The listing builds one solid part. Answer for the finished solid, in the listing's coordinates (mm). A direction names the side the tool comes from. Coordinates: 2 decimals unless noted, no trailing zeros. Order: outer loops, then holes, each group sorted by start corner. A loop starts at its lowest first (then second) coordinate and runs counter-clockwise, first axis right, second up.
```python
from build123d import *

# Parameters (mm, degrees)
BOSS_EXTRUDE1_DEPTH = 139
SKETCH5_R           = 2
CUT_EXTRUDE1_DEPTH  = 148.549991528
SKETCH6_W           = 3
SKETCH6_H           = 35
BOSS_EXTRUDE2_DEPTH = 35
SKETCH7_W           = 133
SKETCH7_H           = 35
BOSS_EXTRUDE3_DEPTH = 5
SKETCH8_W           = 133
SKETCH8_H           = 35
CUT_EXTRUDE2_DEPTH  = 20
SKETCH9_W           = 3
SKETCH9_H           = 12
BOSS_EXTRUDE4_DEPTH = 25
SKETCH10_W          = 133
SKETCH10_H          = 50
BOSS_EXTRUDE5_DEPTH = 20
SKETCH11_W          = 139
SKETCH11_H          = 53
CUT_EXTRUDE3_DEPTH  = 20


with BuildPart() as part:
    # Sketch3 → Boss-Extrude1 (new body)
    with BuildSketch(Plane(origin=(0, 0, 0), x_dir=(0, 0, -1), z_dir=(1, 0, 0))):
        Polygon((-34.8080918, 35), (-34.8080918, 10), (-22.8080918, 10), (-22.8080918, 35), (-19.8080918, 35), (-19.8080918, 0), (15.1919082, 0), (15.1919082, -3), (-29.8080918, -3), (-37.8080918, -3), (-37.8080918, 0), (-37.8080918, 35), align=None)
    extrude(amount=BOSS_EXTRUDE1_DEPTH)

    # Sketch5 → Cut-Extrude1 (cut, through all)
    with BuildSketch(Plane(origin=(0, 0, 19.8080918), x_dir=(-1, 0, 0), z_dir=(0, 0, -1))):
        with Locations(Location((-119, 30, 0), (0, 0, 90))):
            Circle(SKETCH5_R)
        with BuildLine():
            Line((-85, 32), (-15, 32))
            ThreePointArc((-15, 32), (-13, 30), (-15, 28))
            Line((-15, 28), (-85, 28))
            ThreePointArc((-85, 28), (-87, 30), (-85, 32))
        make_face()
    extrude(amount=-CUT_EXTRUDE1_DEPTH, mode=Mode.SUBTRACT)

    # Sketch6 → Boss-Extrude2 (add)
    with BuildSketch(Plane(origin=(0, 0, 0), x_dir=(1, 0, 0), z_dir=(0, 1, 0))):
        with Locations((1.5, -2.3080918)):
            Rectangle(SKETCH6_W, SKETCH6_H)
        with Locations((137.5, -2.3080918)):
            Rectangle(SKETCH6_W, SKETCH6_H)
    extrude(amount=BOSS_EXTRUDE2_DEPTH)

    # Sketch7 → Boss-Extrude3 (add)
    with BuildSketch(Plane(origin=(0, 0, 19.8080918), x_dir=(-1, 0, 0), z_dir=(0, 0, -1))):
        with Locations((-69.5, 17.5)):
            Rectangle(SKETCH7_W, SKETCH7_H)
    extrude(amount=BOSS_EXTRUDE3_DEPTH)

    # Sketch8 → Cut-Extrude2 (cut)
    with BuildSketch(Plane(origin=(0, 0, 14.8080918), x_dir=(-1, 0, 0), z_dir=(0, 0, -1))):
        with Locations((-69.5, 17.5)):
            Rectangle(SKETCH8_W, SKETCH8_H)
    extrude(amount=-CUT_EXTRUDE2_DEPTH, mode=Mode.SUBTRACT)

    # Sketch9 → Boss-Extrude4 (add)
    with BuildSketch(Plane(origin=(0, 10, 0), x_dir=(1, 0, 0), z_dir=(0, 1, 0))):
        with Locations((137.5, -28.8080918)):
            Rectangle(SKETCH9_W, SKETCH9_H)
        with Locations((1.5, -28.8080918)):
            Rectangle(SKETCH9_W, SKETCH9_H)
    extrude(amount=BOSS_EXTRUDE4_DEPTH)

    # Sketch10 → Boss-Extrude5 (add)
    with BuildSketch(Plane(origin=(0, 0, 0), x_dir=(1, 0, 0), z_dir=(0, 1, 0))):
        with Locations((69.5, -9.8080918)):
            Rectangle(SKETCH10_W, SKETCH10_H)
    extrude(amount=BOSS_EXTRUDE5_DEPTH)

    # Sketch11 → Cut-Extrude3 (cut)
    with BuildSketch(Plane.XZ.offset(3)):
        with Locations((69.5, 11.3080918)):
            Rectangle(SKETCH11_W, SKETCH11_H)
    extrude(amount=-CUT_EXTRUDE3_DEPTH, mode=Mode.SUBTRACT)


solid = part.part
```
1) The mould has two halves that part along X. Classify faces 1 (the flat face through (136, 27, 10)), 2 (the flat face through (0, 26, 12)), 3 (the flat face through (139, 26, 12)), 4 (the flat face through (69, 26, 37.808)): released by +X, released by -X, zero draft, split by the parting line, or undercut.
2) Each of these flat-tipped pins is pushed along its axis until it touches: P1, Ø3.5, axis at x = 119, y = 30, coming from the +Z side; P2, Ø2, axis at x = 86, y = 28.5, coming from the -Z side. Where does it stop, or does it pass through?
3) A cutting plane is placed at B-B, the plane x = 119. Write down the section's boundary in (y, z).
4) A cutting plane is placed at A-A, the plane y = 30. Write down the section's boundary in (x, z), plus the area to 3 significant figures.
5) A cutting plane is placed at D-D, the plane z = 33. Write down the section's boundary in (x, y).
6) For faces 5 (the flat face through (69, 35, 37)), 6 (the cylindrical face through (87, 30, 36)), 7 (the flat face through (68.6, 27.6, 34.808)), determine the directions among +Z, -Z, +X, -X, +Y, -Y from which every point of the face is accessible in a straight line to the end or side of a thin tool.
7) A cutting plane is placed at C-C, the plane y = 24.25. Write down the section's boundary in (x, z).
8) Straight lines are drawn through the part: probe 1 along X at (y, z) = (30, 37.2); probe 2 along Y at (x, z) = (20, 35); probe 3 along X at (y, z) = (22, 7). For each, find the intervals that lie inside material, in ascending order.
Working result:
1. face 1: undercut
1. face 2: released by -X
1. face 3: released by +X
1. face 4: zero draft
2. P1: passes through
2. P2: stops at z = 34.81
3. outline: (17, -15.19) - (20, -15.19) - (20, 34.81) - (28, 34.81) - (28, 37.81) - (17, 37.81) - close; (32, 34.81) - (35, 34.81) - (35, 37.81) - (32, 37.81) - close
4. outline: (0, -15.19) - (3, -15.19) - (3, 34.81) - (13, 34.81) - (13, 37.81) - (0, 37.81) - close; (87, 34.81) - (117, 34.81) - (117, 37.81) - (87, 37.81) - close; (121, 34.81) - (136, 34.81) - (136, -15.19) - (139, -15.19) - (139, 37.81) - (121, 37.81) - close
4. area: 483 mm2
5. outline: (0, 17) - (139, 17) - (139, 35) - (136, 35) - (136, 20) - (3, 20) - (3, 35) - (0, 35) - close
6. face 5: +Z, -Z, +X, -X, +Y
6. face 6: +Z, -Z
6. face 7: -Z, +Y
7. outline: (0, -15.19) - (3, -15.19) - (3, 34.81) - (136, 34.81) - (136, -15.19) - (139, -15.19) - (139, 37.81) - (0, 37.81) - close
8. probe 1: x = 0 to 13, 87 to 117, 121 to 139
8. probe 2: y = 17 to 28, 32 to 35
8. probe 3: x = 0 to 3, 136 to 139
